Build history of the part. All positions in model axes, mm. A direction names the side the tool comes from. Coordinates: 2 decimals unless noted, no trailing zeros. Write each loop counter-clockwise with the first axis right and the second up, starting at its lowest first coordinate (ties: lowest second). Pieces come first, ordered by that corner, then holes. Notation, with made-up numbers: (34, -36) -> (67, -36) arc R9 ccw to (67, -28) -> close; hole circle Ø10 at (-27.75, 41). An arc over 180 degrees is marked (long way). Write each question's results on one line, items separated by ' | '. Start each with the question number.
Q1. Saw through at B-B on y = 169.5. Give the cut face in (x, z), and give its area (3 significant figures).
Q2. Drop a flat-ended pin along its axis: pin 1 Ø5 at (x, y) = (7.5, 81.47) entering from -Z. Give the stop position or say it passes through.
Q3. Drill centre lines: line 1 (Z direction, x = 14.45, y = 355.5); line 2 (Z direction, x = 11.25, y = 323.5); line 3 (X direction, y = 45, z = -8.5). Where is each one in solid material? Low to high.
Q4. Saw through at A-A on z = -4.5. Count the separate pieces of the cut face and the enclosed holes in it, and give its area (3 significant figures).
Q5. Saw through at C-C on x = 2.75. Give the cut face in (y, z), and give its area (3 significant figures).
Q6. Tool access for faces 1 (the face through (7, 177, 0)), 2 (the face through (13.9, 177, -7)): list every direction of +Z, -Z, +X, -X, +Y, -Y with a clear straight run to the whole face (end or side of a thin tool).
from build123d import *

# Parameters (mm, degrees)
BOSS_EXTRUDE1_DEPTH       = 360
CUT_EXTRUDE1_REACH        = 3.1
SKETCH2_R                 = 2.25
SKETCH3_R                 = 2.25
CUT_EXTRUDE2_DEPTH        = 1.1
LPATTERN1_COUNT           = 5
LPATTERN1_PITCH           = 25.65625
LPATTERN2_COUNT           = 3
LPATTERN2_PITCH           = 124.1875
LPATTERN2_COPY_1_SKETCH_R = 2.25
LPATTERN2_COPY_1_DEPTH    = 1.1
LPATTERN2_COPY_2_SKETCH_R = 2.25
LPATTERN2_COPY_2_DEPTH    = 1.1
LPATTERN2_COPY_3_SKETCH_R = 2.25
LPATTERN2_COPY_3_DEPTH    = 1.1
LPATTERN2_COPY_4_SKETCH_R = 2.25
LPATTERN2_COPY_4_DEPTH    = 1.1
LPATTERN2_COPY_5_SKETCH_R = 2.25
LPATTERN2_COPY_5_DEPTH    = 1.1
LPATTERN2_COPY_6_SKETCH_R = 2.25
LPATTERN2_COPY_6_DEPTH    = 1.1
LPATTERN2_COPY_7_SKETCH_R = 2.25
LPATTERN2_COPY_7_DEPTH    = 1.1
LPATTERN2_COPY_8_SKETCH_R = 2.25
LPATTERN2_COPY_8_DEPTH    = 1.1


with BuildPart() as part:
    # Sketch1 → Boss-Extrude1 (new body)
    with BuildSketch(Plane(origin=(0, 0, 0), x_dir=(1, 0, 0), z_dir=(0, 1, 0))):
        Polygon((0, 0), (15, 0), (15, 12), (13.9, 12), (13.9, 1.1), (0, 1.1), align=None)
    extrude(amount=BOSS_EXTRUDE1_DEPTH)

    # Sketch2 → Cut-Extrude1 (cut, up to next)
    with BuildSketch(Plane.ZY.offset(-13.9), mode=Mode.PRIVATE) as cut_extrude1_sk1:
        with Locations((-4.5, 329.8125)):
            Circle(SKETCH2_R)
    cut_extrude1_tool1 = extrude(cut_extrude1_sk1.sketch, amount=-CUT_EXTRUDE1_REACH, mode=Mode.PRIVATE) & part.part
    add(cut_extrude1_tool1.solids().sort_by_distance((13.9, 329.8125, -4.5))[0], mode=Mode.SUBTRACT)
    # Sketch2 → Cut-Extrude1 (cut, up to next)
    with BuildSketch(Plane.ZY.offset(-13.9), mode=Mode.PRIVATE) as cut_extrude1_sk2:
        with Locations((-4.5, 304.125)):
            Circle(SKETCH2_R)
    cut_extrude1_tool2 = extrude(cut_extrude1_sk2.sketch, amount=-CUT_EXTRUDE1_REACH, mode=Mode.PRIVATE) & part.part
    add(cut_extrude1_tool2.solids().sort_by_distance((13.9, 304.125, -4.5))[0], mode=Mode.SUBTRACT)
    # Sketch2 → Cut-Extrude1 (cut, up to next)
    with BuildSketch(Plane.ZY.offset(-13.9), mode=Mode.PRIVATE) as cut_extrude1_sk3:
        with Locations((-4.5, 278.4375)):
            Circle(SKETCH2_R)
    cut_extrude1_tool3 = extrude(cut_extrude1_sk3.sketch, amount=-CUT_EXTRUDE1_REACH, mode=Mode.PRIVATE) & part.part
    add(cut_extrude1_tool3.solids().sort_by_distance((13.9, 278.4375, -4.5))[0], mode=Mode.SUBTRACT)
    # Sketch2 → Cut-Extrude1 (cut, up to next)
    with BuildSketch(Plane.ZY.offset(-13.9), mode=Mode.PRIVATE) as cut_extrude1_sk4:
        with Locations((-4.5, 252.75)):
            Circle(SKETCH2_R)
    cut_extrude1_tool4 = extrude(cut_extrude1_sk4.sketch, amount=-CUT_EXTRUDE1_REACH, mode=Mode.PRIVATE) & part.part
    add(cut_extrude1_tool4.solids().sort_by_distance((13.9, 252.75, -4.5))[0], mode=Mode.SUBTRACT)
    # Sketch2 → Cut-Extrude1 (cut, up to next)
    with BuildSketch(Plane.ZY.offset(-13.9), mode=Mode.PRIVATE) as cut_extrude1_sk5:
        with Locations((-4.5, 231.375)):
            Circle(SKETCH2_R)
    cut_extrude1_tool5 = extrude(cut_extrude1_sk5.sketch, amount=-CUT_EXTRUDE1_REACH, mode=Mode.PRIVATE) & part.part
    add(cut_extrude1_tool5.solids().sort_by_distance((13.9, 231.375, -4.5))[0], mode=Mode.SUBTRACT)
    # Sketch2 → Cut-Extrude1 (cut, up to next)
    with BuildSketch(Plane.ZY.offset(-13.9), mode=Mode.PRIVATE) as cut_extrude1_sk6:
        with Locations((-4.5, 205.6875)):
            Circle(SKETCH2_R)
    cut_extrude1_tool6 = extrude(cut_extrude1_sk6.sketch, amount=-CUT_EXTRUDE1_REACH, mode=Mode.PRIVATE) & part.part
    add(cut_extrude1_tool6.solids().sort_by_distance((13.9, 205.6875, -4.5))[0], mode=Mode.SUBTRACT)
    # Sketch2 → Cut-Extrude1 (cut, up to next)
    with BuildSketch(Plane.ZY.offset(-13.9), mode=Mode.PRIVATE) as cut_extrude1_sk7:
        with Locations((-4.5, 180)):
            Circle(SKETCH2_R)
    cut_extrude1_tool7 = extrude(cut_extrude1_sk7.sketch, amount=-CUT_EXTRUDE1_REACH, mode=Mode.PRIVATE) & part.part
    add(cut_extrude1_tool7.solids().sort_by_distance((13.9, 180, -4.5))[0], mode=Mode.SUBTRACT)
    # Sketch2 → Cut-Extrude1 (cut, up to next)
    with BuildSketch(Plane.ZY.offset(-13.9), mode=Mode.PRIVATE) as cut_extrude1_sk8:
        with Locations((-4.5, 154.3125)):
            Circle(SKETCH2_R)
    cut_extrude1_tool8 = extrude(cut_extrude1_sk8.sketch, amount=-CUT_EXTRUDE1_REACH, mode=Mode.PRIVATE) & part.part
    add(cut_extrude1_tool8.solids().sort_by_distance((13.9, 154.3125, -4.5))[0], mode=Mode.SUBTRACT)
    # Sketch2 → Cut-Extrude1 (cut, up to next)
    with BuildSketch(Plane.ZY.offset(-13.9), mode=Mode.PRIVATE) as cut_extrude1_sk9:
        with Locations((-4.5, 128.625)):
            Circle(SKETCH2_R)
    cut_extrude1_tool9 = extrude(cut_extrude1_sk9.sketch, amount=-CUT_EXTRUDE1_REACH, mode=Mode.PRIVATE) & part.part
    add(cut_extrude1_tool9.solids().sort_by_distance((13.9, 128.625, -4.5))[0], mode=Mode.SUBTRACT)
    # Sketch2 → Cut-Extrude1 (cut, up to next)
    with BuildSketch(Plane.ZY.offset(-13.9), mode=Mode.PRIVATE) as cut_extrude1_sk10:
        with Locations((-4.5, 107.25)):
            Circle(SKETCH2_R)
    cut_extrude1_tool10 = extrude(cut_extrude1_sk10.sketch, amount=-CUT_EXTRUDE1_REACH, mode=Mode.PRIVATE) & part.part
    add(cut_extrude1_tool10.solids().sort_by_distance((13.9, 107.25, -4.5))[0], mode=Mode.SUBTRACT)
    # Sketch2 → Cut-Extrude1 (cut, up to next)
    with BuildSketch(Plane.ZY.offset(-13.9), mode=Mode.PRIVATE) as cut_extrude1_sk11:
        with Locations((-4.5, 81.5625)):
            Circle(SKETCH2_R)
    cut_extrude1_tool11 = extrude(cut_extrude1_sk11.sketch, amount=-CUT_EXTRUDE1_REACH, mode=Mode.PRIVATE) & part.part
    add(cut_extrude1_tool11.solids().sort_by_distance((13.9, 81.5625, -4.5))[0], mode=Mode.SUBTRACT)
    # Sketch2 → Cut-Extrude1 (cut, up to next)
    with BuildSketch(Plane.ZY.offset(-13.9), mode=Mode.PRIVATE) as cut_extrude1_sk12:
        with Locations((-4.5, 55.875)):
            Circle(SKETCH2_R)
    cut_extrude1_tool12 = extrude(cut_extrude1_sk12.sketch, amount=-CUT_EXTRUDE1_REACH, mode=Mode.PRIVATE) & part.part
    add(cut_extrude1_tool12.solids().sort_by_distance((13.9, 55.875, -4.5))[0], mode=Mode.SUBTRACT)
    # Sketch2 → Cut-Extrude1 (cut, up to next)
    with BuildSketch(Plane.ZY.offset(-13.9), mode=Mode.PRIVATE) as cut_extrude1_sk13:
        with Locations((-4.5, 30.1875)):
            Circle(SKETCH2_R)
    cut_extrude1_tool13 = extrude(cut_extrude1_sk13.sketch, amount=-CUT_EXTRUDE1_REACH, mode=Mode.PRIVATE) & part.part
    add(cut_extrude1_tool13.solids().sort_by_distance((13.9, 30.1875, -4.5))[0], mode=Mode.SUBTRACT)
    # Sketch2 → Cut-Extrude1 (cut, up to next)
    with BuildSketch(Plane.ZY.offset(-13.9), mode=Mode.PRIVATE) as cut_extrude1_sk14:
        with Locations((-4.5, 4.5)):
            Circle(SKETCH2_R)
    cut_extrude1_tool14 = extrude(cut_extrude1_sk14.sketch, amount=-CUT_EXTRUDE1_REACH, mode=Mode.PRIVATE) & part.part
    add(cut_extrude1_tool14.solids().sort_by_distance((13.9, 4.5, -4.5))[0], mode=Mode.SUBTRACT)
    # Sketch2 → Cut-Extrude1 (cut, up to next)
    with BuildSketch(Plane.ZY.offset(-13.9), mode=Mode.PRIVATE) as cut_extrude1_sk15:
        with Locations((-4.5, 355.5)):
            Circle(SKETCH2_R)
    cut_extrude1_tool15 = extrude(cut_extrude1_sk15.sketch, amount=-CUT_EXTRUDE1_REACH, mode=Mode.PRIVATE) & part.part
    add(cut_extrude1_tool15.solids().sort_by_distance((13.9, 355.5, -4.5))[0], mode=Mode.SUBTRACT)

    # Sketch3 → Cut-Extrude2 (cut)
    with BuildSketch(Plane.XY):
        with Locations((7.5, 355.5)):
            Circle(SKETCH3_R)
    cut_extrude2 = extrude(amount=-CUT_EXTRUDE2_DEPTH, mode=Mode.SUBTRACT)

    # LPattern1: Cut-Extrude2 ×5
    with Locations(*[(0, -i * LPATTERN1_PITCH, 0) for i in range(1, LPATTERN1_COUNT)]):
        add(cut_extrude2, mode=Mode.SUBTRACT)

    # LPattern2: Cut-Extrude2 ×3
    with Locations(*[(0, -i * LPATTERN2_PITCH, 0) for i in range(1, LPATTERN2_COUNT)]):
        add(cut_extrude2, mode=Mode.SUBTRACT)

    # LPattern2 copy 1 sketch → LPattern2 copy 1 (cut)
    with BuildSketch(Plane(origin=(0, -149.84375, 0), x_dir=(1, 0, 0), z_dir=(0, 0, 1))):
        with Locations((7.5, 355.5)):
            Circle(LPATTERN2_COPY_1_SKETCH_R)
    extrude(amount=-LPATTERN2_COPY_1_DEPTH, mode=Mode.SUBTRACT)

    # LPattern2 copy 2 sketch → LPattern2 copy 2 (cut)
    with BuildSketch(Plane(origin=(0, -274.03125, 0), x_dir=(1, 0, 0), z_dir=(0, 0, 1))):
        with Locations((7.5, 355.5)):
            Circle(LPATTERN2_COPY_2_SKETCH_R)
    extrude(amount=-LPATTERN2_COPY_2_DEPTH, mode=Mode.SUBTRACT)

    # LPattern2 copy 3 sketch → LPattern2 copy 3 (cut)
    with BuildSketch(Plane(origin=(0, -175.5, 0), x_dir=(1, 0, 0), z_dir=(0, 0, 1))):
        with Locations((7.5, 355.5)):
            Circle(LPATTERN2_COPY_3_SKETCH_R)
    extrude(amount=-LPATTERN2_COPY_3_DEPTH, mode=Mode.SUBTRACT)

    # LPattern2 copy 4 sketch → LPattern2 copy 4 (cut)
    with BuildSketch(Plane(origin=(0, -299.6875, 0), x_dir=(1, 0, 0), z_dir=(0, 0, 1))):
        with Locations((7.5, 355.5)):
            Circle(LPATTERN2_COPY_4_SKETCH_R)
    extrude(amount=-LPATTERN2_COPY_4_DEPTH, mode=Mode.SUBTRACT)

    # LPattern2 copy 5 sketch → LPattern2 copy 5 (cut)
    with BuildSketch(Plane(origin=(0, -201.15625, 0), x_dir=(1, 0, 0), z_dir=(0, 0, 1))):
        with Locations((7.5, 355.5)):
            Circle(LPATTERN2_COPY_5_SKETCH_R)
    extrude(amount=-LPATTERN2_COPY_5_DEPTH, mode=Mode.SUBTRACT)

    # LPattern2 copy 6 sketch → LPattern2 copy 6 (cut)
    with BuildSketch(Plane(origin=(0, -325.34375, 0), x_dir=(1, 0, 0), z_dir=(0, 0, 1))):
        with Locations((7.5, 355.5)):
            Circle(LPATTERN2_COPY_6_SKETCH_R)
    extrude(amount=-LPATTERN2_COPY_6_DEPTH, mode=Mode.SUBTRACT)

    # LPattern2 copy 7 sketch → LPattern2 copy 7 (cut)
    with BuildSketch(Plane(origin=(0, -226.8125, 0), x_dir=(1, 0, 0), z_dir=(0, 0, 1))):
        with Locations((7.5, 355.5)):
            Circle(LPATTERN2_COPY_7_SKETCH_R)
    extrude(amount=-LPATTERN2_COPY_7_DEPTH, mode=Mode.SUBTRACT)

    # LPattern2 copy 8 sketch → LPattern2 copy 8 (cut)
    with BuildSketch(Plane(origin=(0, -351, 0), x_dir=(1, 0, 0), z_dir=(0, 0, 1))):
        with Locations((7.5, 355.5)):
            Circle(LPATTERN2_COPY_8_SKETCH_R)
    extrude(amount=-LPATTERN2_COPY_8_DEPTH, mode=Mode.SUBTRACT)


solid = part.part
Returned:
1) outline: (0, -1.1) -> (13.9, -1.1) -> (13.9, -12) -> (15, -12) -> (15, 0) -> (0, 0) -> close | area: 28.5 mm2
2) pin 1: stops at z = -1.1
3) line 1: z = -12 to -6.75, -2.25 to 0 | line 2: z = -1.1 to 0 | line 3: x = 13.9 to 15
4) separate pieces: 16 | enclosed holes: 0 | area: 322 mm2
5) outline: (0, -1.1) -> (360, -1.1) -> (360, 0) -> (0, 0) -> close | area: 396 mm2
6) face 1: +Z, +X, -X, +Y, -Y | face 2: -Z, -X, +Y, -Y
